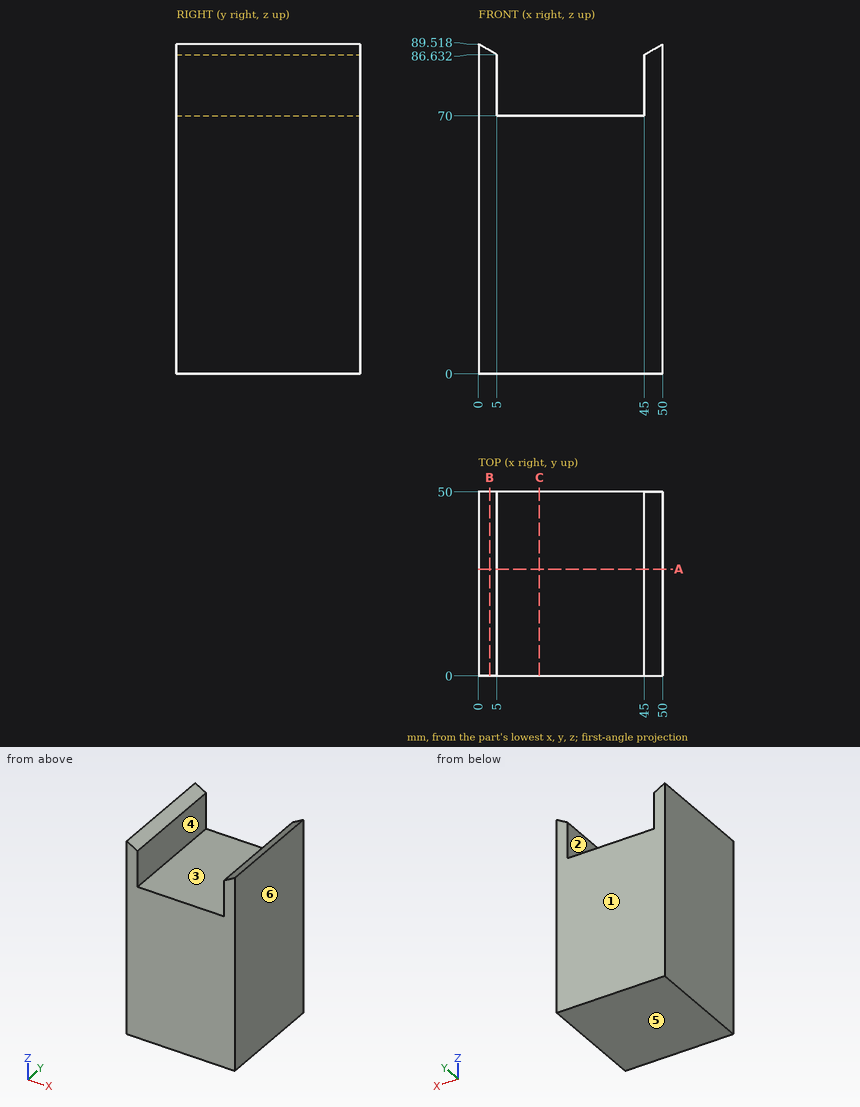
Print and shaded views of the part. All mm, measured from the part's lowest x, y and z. A direction names the side the tool comes from. Give positions to 0.01 mm unless a question says otherwise; leave off trailing zeros. Loops run counter-clockwise (first coordinate to the right, second up) from the corner with the lowest first, then second, coordinate; pieces in that order, holes last. Notation, with made-up numbers: (25.25, 1) - (71.25, 1) arc R27 cw to (71.25, 27) - close; hole circle Ø7 at (76.5, 15). An arc over 180 degrees is marked (long way). Use a Markdown table: item, result.
(1) Wall check: line 1 along Z through (x, y) = (13, 4); line 2 along X through (y, z) = (25.5, 75). Give the ranges that are in metal, low to high.
Taken from the geometry:
| item | result |
|---|---|
| line 1 | 0 to 70 |
| line 2 | 0 to 5, 45 to 50 |
(2) Band-saw the part on C-C (x = 16.5). Give the cut face in (y, z).
Taken from the geometry:
| item | result |
|---|---|
| outline | (0, 0) - (50, 0) - (50, 70) - (0, 70) - close |
(3) Pull direction X, two halves, no side cores. Call the marked faces 3, 4, 5 and 6: +X half, -X half, draft (parallel to the pull), parting line (faces both ways), or undercut.
Taken from the geometry:
| item | result |
|---|---|
| face 3 | undercut |
| face 4 | undercut |
| face 5 | draft |
| face 6 | +X half |
(4) Which spindle directions (+Z, -Z, +X, -X, +Y, -Y) get a long thin tool onto all of the face, cutting with end or side? Do the marked faces 1 and 2. Say none if no direction does.
Taken from the geometry:
| item | result |
|---|---|
| face 1 | +Z, -Z, +X, -X, +Y |
| face 2 | +Z, +Y, -Y |
(5) Band-saw the part on B-B (x = 3). Give the cut face in (y, z).
Taken from the geometry:
| item | result |
|---|---|
| outline | (0, 0) - (50, 0) - (50, 87.79) - (0, 87.79) - close |
(6) Drop flat-ended pins along their axis: pin 1 Ø3 at (x, y) = (5, 34.5) entering from +Z; pin 2 Ø20 at (x, y) = (34.5, 28) entering from +Z. Give the stop position or say it passes through.
Taken from the geometry:
| item | result |
|---|---|
| pin 1 | z = 87.5 |
| pin 2 | z = 70 |
(7) Band-saw the part on A-A (y = 29). Give the cut face in (x, z).
Taken from the geometry:
| item | result |
|---|---|
| outline | (0, 0) - (50, 0) - (50, 89.52) - (45, 86.63) - (45, 70) - (5, 70) - (5, 86.63) - (0, 89.52) - close |
